Source: three-view drawing plus pictorial views. Frame: mm from the lowest corner of the part. A direction names the side the tool comes from. Give positions to 0.01 mm unless a question says otherwise; leave off trailing zeros. Write each loop counter-clockwise with the first axis right and the second up, starting at its lowest first coordinate (ties: lowest second). Pieces come first, ordered by that corner, then holes.
Q1. Pin query (flat end, axial travel): pin 1 (3 mm diameter, centred on x = 2.5, y = 15, fed in from -Z); pin 2 (3 mm diameter, centred on x = 1, y = 37, fed in from +Z); pin 3 (2 mm diameter, centred on y = 34, z = 2, fed in from +X). Return the tip coordinate at first contact, or that it passes through.
Q2. Reachability of the marked faces 1 and 2 from +Z, -Z, +X, -X, +Y, -Y: full face, straight path, thin tool, end or side. Return the list, or none.
Q3. Cut plane C-C on y = 18.5. Return the cut outline in (x, z).
Q4. Cut plane A-A on x = 2.5. Return the cut outline in (y, z), plus the area to 3 significant figures.
Q5. Cut plane B-B on z = 2.5. Return the cut outline in (x, y).
Q6. Line query: L1, parallel to Y at x = 1.95, z = 1.2; L2, parallel to Z at x = 1.75, y = 24; L3, parallel to Z at x = 1.9, y = 19.5. Output: solid intervals per line, ascending.
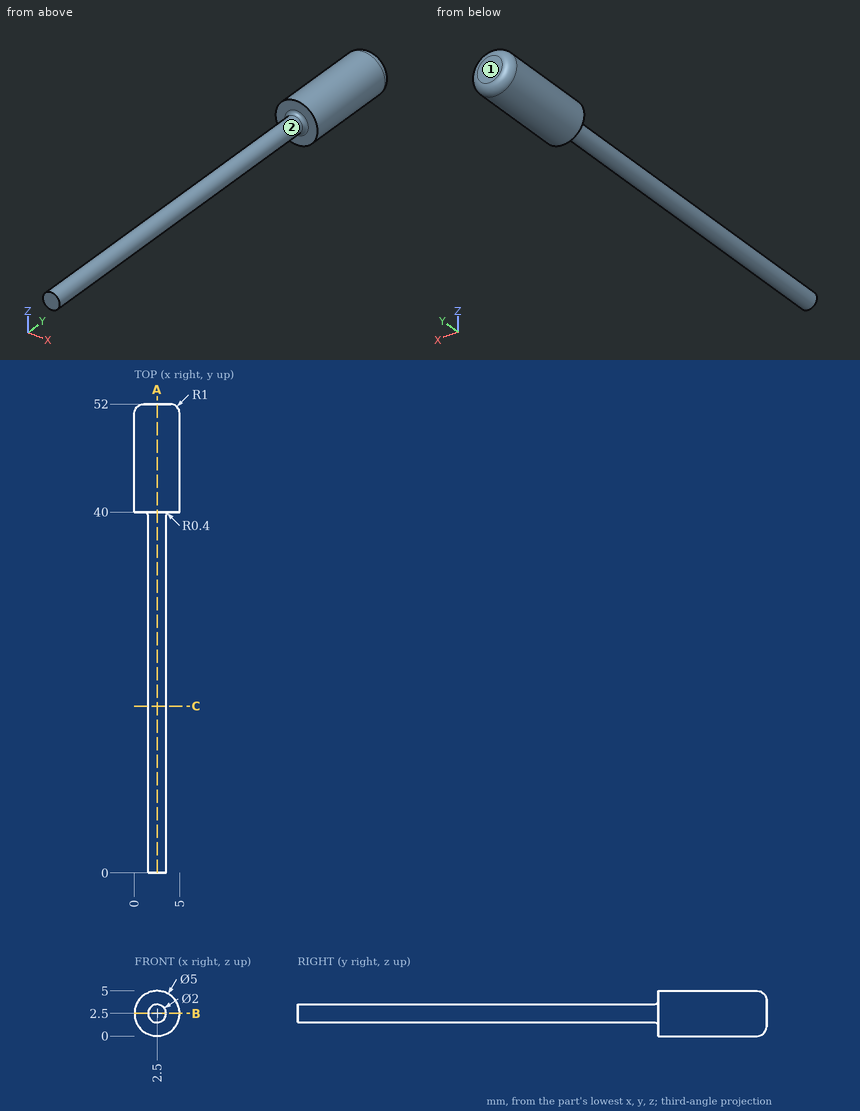
Data:
1. pin 1: stops at z = 1.5
1. pin 2: stops at z = 3.5
1. pin 3: stops at x = 3.5
2. face 1: +Z, -Z, +X, -X, +Y
2. face 2: -Y
3. outline: circle Ø2 at (2.5, 2.5)
4. outline: (0, 1.5) - (39.6, 1.5) arc R0.4 cw to (40, 1.1) - (40, 0) - (51, 0) arc R1 ccw to (52, 1) - (52, 4) arc R1 ccw to (51, 5) - (40, 5) - (40, 3.9) arc R0.4 cw to (39.6, 3.5) - (0, 3.5) - close
4. area: 140 mm2
5. outline: (0, 40) - (1.1, 40) arc R0.4 cw to (1.5, 39.6) - (1.5, 0) - (3.5, 0) - (3.5, 39.6) arc R0.4 cw to (3.9, 40) - (5, 40) - (5, 51) arc R1 ccw to (4, 52) - (1, 52) arc R1 ccw to (0, 51) - close
6. L1: y = 40 to 52
6. L2: z = 1.84 to 3.16
6. L3: z = 1.7 to 3.3
